Check sheet for the modelled part. Datum: model origin and axes. Units: mm. A direction names the side the tool comes from. Give positions to 0.01 mm unless a question says otherwise; leave off trailing zeros. Order: outer loops, then holes, each group sorted by start corner. A loop starts at its lowest first (then second) coordinate and runs counter-clockwise, first axis right, second up.
```python
from build123d import *

# Parameters (mm, degrees)
SKETCH_1_R               = 75
SKETCH_1_R_2             = 1.4
SKETCH_1_R_3             = 13.5
EXTRUDE_1_DEPTH          = 3
SKETCH_2_R               = 57.5
SKETCH_2_R_2             = 50
EXTRUDE_3_DEPTH          = 80
CUT_EXTRUDE_1_DEPTH      = 80
CUT_EXTRUDE_1_DEPTH_BACK = 80
SKETCH_4_W               = 50
SKETCH_4_H               = 40
CUT_EXTRUDE_START        = -80
SKETCH_5_R               = 75
SKETCH_5_R_2             = 57.5
CUT_EXTRUDE_2_DEPTH      = 80


with BuildPart() as part:
    # Sketch 1 → Extrude 1 (new body)
    with BuildSketch(Plane(origin=(0, 0, 0), x_dir=(1, 0, 0), z_dir=(0, 1, 0))):
        with Locations(Location((0, 0, 0), (0, 0, 270))):
            Circle(SKETCH_1_R)
        with Locations(Location((11.5, 11.5, 0), (0, 0, 270))):
            Circle(SKETCH_1_R_2, mode=Mode.SUBTRACT)
        with Locations(Location((-11.5, 11.5, 0), (0, 0, 270))):
            Circle(SKETCH_1_R_2, mode=Mode.SUBTRACT)
        with Locations(Location((-11.5, -11.5, 0), (0, 0, 270))):
            Circle(SKETCH_1_R_2, mode=Mode.SUBTRACT)
        with Locations(Location((11.5, -11.5, 0), (0, 0, 270))):
            Circle(SKETCH_1_R_2, mode=Mode.SUBTRACT)
        with Locations(Location((0, 0, 0), (0, 0, 270))):
            Circle(SKETCH_1_R_3, mode=Mode.SUBTRACT)
    extrude(amount=EXTRUDE_1_DEPTH)

    # Sketch 2 → Extrude 3 (add)
    with BuildSketch(Plane(origin=(0, 3, 0), x_dir=(1, 0, 0), z_dir=(0, 1, 0))):
        with Locations(Location((0, 0, 0), (0, 0, 270))):
            Circle(SKETCH_2_R)
        with Locations(Location((0, 0, 0), (0, 0, 270))):
            Circle(SKETCH_2_R_2, mode=Mode.SUBTRACT)
    extrude(amount=EXTRUDE_3_DEPTH)

    # Sketch 4 → Cut-Extrude 1 (cut, two sides: drawn at the far end of the back side and taken through both)
    with BuildSketch(Plane.XY.offset(-CUT_EXTRUDE_1_DEPTH_BACK)):
        with Locations((0, 83)):
            Rectangle(SKETCH_4_W, SKETCH_4_H)
    extrude(amount=CUT_EXTRUDE_1_DEPTH + CUT_EXTRUDE_1_DEPTH_BACK, mode=Mode.SUBTRACT)

    # Sketch 5 → Cut-Extrude 2 (cut)
    with BuildSketch(Plane(origin=(0, 3, 0), x_dir=(1, 0, 0), z_dir=(0, 1, 0)).offset(CUT_EXTRUDE_START)):
        Circle(SKETCH_5_R)
        with Locations(Location((0, 0, 0), (0, 0, 64.228538259))):
            Circle(SKETCH_5_R_2, mode=Mode.SUBTRACT)
    extrude(amount=CUT_EXTRUDE_2_DEPTH, mode=Mode.SUBTRACT)


solid = part.part
```
(1) Material ranges on L1, parallel to X at y = 1.4, z = 11.5; L2, parallel to X at y = 1, z = -11; L3, parallel to X at y = 0.8, z = 0, recorded low to high.
Response values:
L1: x = -56.34 to -12.9, -10.1 to -7.07, 7.07 to 10.1, 12.9 to 56.34
L2: x = -56.44 to -12.81, -10.19 to -7.83, 7.83 to 10.19, 12.81 to 56.44
L3: x = -57.5 to -13.5, 13.5 to 57.5
(2) Set-up check for faces 4 (the face through (-51, 83, 0)), 5 (the face through (-10, 3, 10)), 6 (the face through (25, 73, -48)): record each of +Z, -Z, +X, -X, +Y, -Y from which the full face is reachable in a straight line by a thin tool's end or side.
Response values:
face 4: +Z, -Z, +X, -X, +Y
face 5: +Y
face 6: +Z, -Z, +Y
(3) Gauge pin test, flat ends, axial feed: pin 1 Ø12 at (x, z) = (-6.5, 41.5) entering from +Y; pin 2 Ø2.5 at (y, z) = (73, -48.5) entering from -X; pin 3 Ø10 at (x, y) = (-20.5, 43.5) entering from -Z. Record the tip position at first contact, or that the pin passes through.
Response values:
pin 1: stops at y = 3
pin 2: stops at x = -32.77
pin 3: stops at z = -55.37
(4) Cross-section at B-B on x = -28. Enter the section's corners in (y, z), then the cut area to 3 significant figures.
Response values:
outline: (0, -50.22) - (83, -50.22) - (83, -41.42) - (3, -41.42) - (3, 41.42) - (83, 41.42) - (83, 50.22) - (0, 50.22) - close
area: 1,710 mm2
(5) Cross-section at A-A on y = 37.5. Enter the section's corners in (x, z), then the cut area to 3 significant figures.
Response values:
outline: circle Ø115 at (0, 0); hole circle Ø100 at (0, 0)
area: 2,530 mm2
(6) Release check for a two-part mould opening along X. For faces 1 (the face through (-25, 73, 47)), 2 (the face through (56.955, 40.919, 7.898)), 3 (the face through (14, 0, -1)) record: released by +X, released by -X, zero draft, split by the parting line, or undercut.
Response values:
face 1: undercut
face 2: split by the parting line
face 3: zero draft
